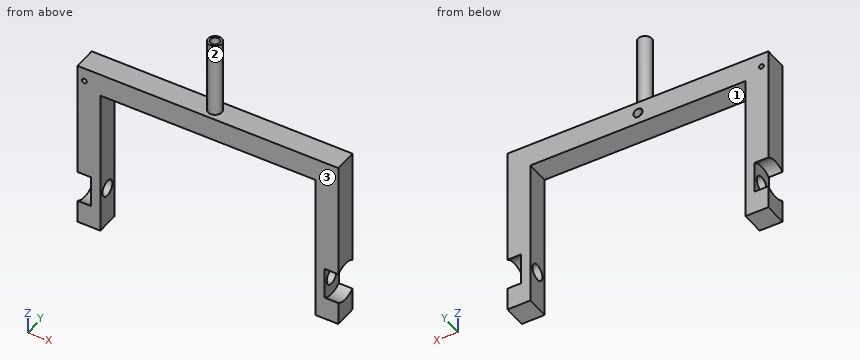
```python
from build123d import *

# Parameters (mm, degrees)
BOSS_EXTRUDE1_DEPTH = 10
SKETCH2_R           = 8.55
CUT_EXTRUDE1_DEPTH  = 6
SKETCH3_R           = 3.5
CUT_EXTRUDE2_DEPTH  = 127.447617613
SKETCH4_R           = 3
BOSS_EXTRUDE2_DEPTH = 33
SKETCH5_R           = 1.05
CUT_EXTRUDE3_DEPTH  = 88.028730888
SKETCH6_R           = 2
CUT_EXTRUDE4_DEPTH  = 38
SKETCH7_R           = 2
CUT_EXTRUDE5_DEPTH  = 5
FILLET2_R           = 6


with BuildPart() as part:
    # Sketch1 → Boss-Extrude1 (new body)
    with BuildSketch(Plane(origin=(0, 0, 0), x_dir=(1, 0, 0), z_dir=(0, 1, 0))):
        Polygon((-47, 0), (47, 0), (47, 65), (57, 65), (57, -10), (-57, -10), (-57, 65), (-47, 65), align=None)
    extrude(amount=BOSS_EXTRUDE1_DEPTH)

    # Sketch2 → Cut-Extrude1 (cut)
    with BuildSketch(Plane(origin=(57, 0, 0), x_dir=(0, 0, -1), z_dir=(1, 0, 0))):
        with Locations((48, 5)):
            Circle(SKETCH2_R)
    cut_extrude1 = extrude(amount=-CUT_EXTRUDE1_DEPTH, mode=Mode.SUBTRACT)

    # Mirror1: Cut-Extrude1 across plane
    add(cut_extrude1.mirror(Plane(origin=(0, 0, 0), x_dir=(0, 0, 1), z_dir=(1, 0, 0))), mode=Mode.SUBTRACT)

    # Sketch3 → Cut-Extrude2 (cut, through all)
    with BuildSketch(Plane(origin=(51, 0, 0), x_dir=(0, 0, -1), z_dir=(1, 0, 0))):
        with Locations(Location((48, 5, 0), (0, 0, 180))):
            Circle(SKETCH3_R)
    extrude(amount=-CUT_EXTRUDE2_DEPTH, mode=Mode.SUBTRACT)

    # Sketch4 → Boss-Extrude2 (add)
    with BuildSketch(Plane.XY.offset(10)):
        with Locations(Location((0, 5, 0), (0, 0, 180))):
            Circle(SKETCH4_R)
    extrude(amount=BOSS_EXTRUDE2_DEPTH)

    # Sketch5 → Cut-Extrude3 (cut, through all)
    with BuildSketch(Plane(origin=(0, 10, 0), x_dir=(1, 0, 0), z_dir=(0, 1, 0))):
        with Locations(Location((-54, -4, 0), (0, 0, 270))):
            Circle(SKETCH5_R)
    extrude(amount=-CUT_EXTRUDE3_DEPTH, mode=Mode.SUBTRACT)

    # Sketch6 → Cut-Extrude4 (cut)
    with BuildSketch(Plane.XY.offset(43)):
        with Locations((0, 5)):
            Circle(SKETCH6_R)
    extrude(amount=-CUT_EXTRUDE4_DEPTH, mode=Mode.SUBTRACT)

    # Sketch7 → Cut-Extrude5 (cut)
    with BuildSketch(Plane(origin=(0, 10, 0), x_dir=(1, 0, 0), z_dir=(0, 1, 0))):
        with Locations(Location((0, -5, 0), (0, 0, 270))):
            Circle(SKETCH7_R)
    extrude(amount=-CUT_EXTRUDE5_DEPTH, mode=Mode.SUBTRACT)

    # Fillet2
    # the kernel refuses this fillet: 6 mm, written as the material it takes off along each edge
    with BuildSketch(Plane(origin=(17, 5, 5), x_dir=(0, 0, -1), z_dir=(-1, 0, 0))) as fillet2_piece_1_section:
        with BuildLine():
            CenterArc((FILLET2_R, FILLET2_R), FILLET2_R, 180, 90)
            Line((0, FILLET2_R), (0, 0))
            Line((0, 0), (FILLET2_R, 0))
        make_face()
    fillet2_piece_1 = extrude(amount=34, mode=Mode.PRIVATE)
    fillet2_piece_1 = fillet2_piece_1 & Plane(origin=(0, 4.127189323, 5), x_dir=(0, 0, 1), z_dir=(0, 1, 0)) * Cylinder(2, 92, mode=Mode.PRIVATE)
    fillet2_piece_1 = fillet2_piece_1 & Plane(origin=(0, 5, 4.127189323), x_dir=(1, 0, 0), z_dir=(0, 0, 1)) * Cylinder(2, 92, mode=Mode.PRIVATE)
    add(fillet2_piece_1, mode=Mode.SUBTRACT)


solid = part.part
```
Work out the finished part from the listing and answer in its coordinate system (mm). Face numbers are marked on the shaded views. Give positions to 0.01 mm unless a question says otherwise; leave off trailing zeros. Loops run counter-clockwise (first coordinate to the right, second up) from the corner with the lowest first, then second, coordinate; pieces in that order, holes last. Notation, with made-up numbers: (85, -23) -> (130, -23) arc R13 cw to (130, -15) -> close; hole circle Ø5 at (69.25, 76.25). An arc over 180 degrees is marked (long way). One line per question, with ' | ' between items. Start each with the question number.
1) Section B-B, the plane z = -21 is taken. Determine the outline of the cut face in (x, y), then the cut area to 3 significant figures.
2) Section A-A, the plane y = 5 is taken. State how many separate pieces and enclosed holes the cut face has, then the cut area to 3 significant figures.
3) Each of these flat-tipped pins is pushed along its axis until it touches: pin 1 (5 mm diameter, centred on x = -19.5, y = 4, fed in from +Z); pin 2 (1.3 mm diameter, centred on x = -54, z = 4, fed in from -Y); pin 3 (5 mm diameter, centred on x = 0, y = 5, fed in from -Z); pin 4 (1 mm diameter, centred on y = 1, z = -52, fed in from +X). Where does it stop, or does it pass through?
4) Section C-C, the plane z = -48 is taken. Determine the outline of the cut face in (x, y), then the cut area to 3 significant figures.
5) Section D-D, the plane x = -29 is taken. Determine the outline of the cut face in (y, z), then the cut area to 3 significant figures.
6) Straight lines are drawn through the part: L1, parallel to Z at x = -48.2, y = 5; L2, parallel to X at y = 3.25, z = -28; L3, parallel to X at y = 8.75, z = -45. For each, find the intervals that lie inside material, in ascending order.
7) Determine the mould class of the marked faces 1, 2 and 3 for opening direction X: +X half, -X half, draft (parallel to the pull), parting line (faces both ways), or undercut.
Resolved:
1) outline: (-57, 0) -> (-47, 0) -> (-47, 10) -> (-57, 10) -> close; (47, 0) -> (57, 0) -> (57, 10) -> (47, 10) -> close | area: 200 mm2
2) separate pieces: 3 | enclosed holes: 1 | area: 2,220 mm2
3) pin 1: z = 10 | pin 2: through | pin 3: z = 0 | pin 4: x = 51
4) outline: (-51, 0) -> (-47, 0) -> (-47, 1.5) -> (-51, 1.5) -> close; (-51, 8.5) -> (-47, 8.5) -> (-47, 10) -> (-51, 10) -> close; (47, 0) -> (51, 0) -> (51, 1.5) -> (47, 1.5) -> close; (47, 8.5) -> (51, 8.5) -> (51, 10) -> (47, 10) -> close | area: 24.0 mm2
5) outline: (0, 0) -> (10, 0) -> (10, 10) -> (0, 10) -> close | area: 100 mm2
6) L1: -65 to -51.5, -44.5 to 10 | L2: -57 to -47, 47 to 57 | L3: -51 to -47, 47 to 51
7) face 1: undercut | face 2: parting line | face 3: draft
